Input: part model. Units: mm. Frame: model coordinates. A direction names the side the tool comes from. Give positions to 0.01 mm unless a question says otherwise; leave off trailing zeros. Loops run counter-clockwise (first coordinate to the right, second up) from the corner with the lowest first, then second, coordinate; pieces in that order, holes last. Notation, with made-up numbers: (-19.75, 53) -> (0.25, 53) arc R13 cw to (0.25, 62) -> close; hole circle Ø6 at (35.25, 51.5). An arc over 180 degrees is marked (long way). Answer as a JSON object with one key per item and string values.
```python
from build123d import *

# Parameters (mm, degrees)
F0_W     = 95
F0_H     = 90
F1_DEPTH = 20
F2_R     = 32.5
F3_DEPTH = 25
F4_R     = 17.5
F5_DEPTH = 25


with BuildPart() as f1:
    # F0 (on Top) → F1 (new body)
    with BuildSketch(Plane.XY):
        with Locations((-1.046643, 7.062163)):
            Rectangle(F0_W, F0_H)
        with BuildLine():
            ThreePointArc((46.453357, -37.937837), (91.453357, 7.062163), (46.453357, 52.062163))
            Line((46.453357, 52.062163), (46.453357, -37.937837))
        make_face()
    extrude(amount=F1_DEPTH)

    # F2 (on face) → F3 (join)
    with BuildSketch(Plane.XY.offset(20)):
        with Locations((46.453357, 7.062163)):
            Circle(F2_R)
    extrude(amount=F3_DEPTH)

    # F4 (on face) → F5 (cut)
    with BuildSketch(Plane.XY.offset(45)):
        with Locations((46.453357, 7.062163)):
            Circle(F4_R)
    extrude(amount=-F5_DEPTH, mode=Mode.SUBTRACT)


solid = f1.part
```
Q1. Section B-B, the plane x = 15.5. Return the cut outline in (y, z).
Evaluation:
{"outline": "(-37.94, 0) -> (52.06, 0) -> (52.06, 20) -> (16.97, 20) -> (16.97, 45) -> (-2.84, 45) -> (-2.84, 20) -> (-37.94, 20) -> close"}
Q2. Access query for faces 1 (the cylindrical face through (28.97, 7.83, 32.67)), 2 (the cylindrical face through (91.442, 6.073, 9.86)). Directions: +Z, -Z, +X, -X, +Y, -Y. A direction counts if a zero-diameter tool reaches every point of the face in a straight line with its end or side. Return the directions, or none.
Evaluation:
{"face 1": "+Z", "face 2": "+Z, -Z, +X"}
Q3. Section D-D, the plane z = 17.5. Return the cut outline in (x, y).
Evaluation:
{"outline": "(-48.55, -37.94) -> (46.45, -37.94) arc R45 ccw to (46.45, 52.06) -> (-48.55, 52.06) -> close"}
Q4. Pin query (flat end, axial travel): pin 1 (17.5 mm diameter, centred on x = 43.5, y = 3.5, fed in from +Z); pin 2 (1.5 mm diameter, centred on x = -26, z = 22, fed in from +Y); pin 3 (1 mm diameter, centred on x = 63, z = 24, fed in from -Y); pin 4 (2 mm diameter, centred on y = -1, z = 12.5, fed in from +X). Return the tip coordinate at first contact, or that it passes through.
Evaluation:
{"pin 1": "stops at z = 20", "pin 2": "passes through", "pin 3": "stops at y = -21.2", "pin 4": "stops at x = 90.9"}
Q5. Section A-A, the plane y = -18.5. Return the cut outline in (x, z).
Evaluation:
{"outline": "(-48.55, 0) -> (83.49, 0) -> (83.49, 20) -> (66.52, 20) -> (66.52, 45) -> (26.38, 45) -> (26.38, 20) -> (-48.55, 20) -> close"}
Q6. Ray query, line 1 along X through (y, z) = (7, 37); line 2 along Z through (x, y) = (46, 9); line 3 along Y through (x, z) = (44, 24.5). Return the intervals inside material, ascending.
Evaluation:
{"line 1": "x = 13.95 to 28.95, 63.95 to 78.95", "line 2": "z = 0 to 20", "line 3": "y = -25.35 to -10.27, 24.39 to 39.47"}
Q7. Draft query along Y for faces 3 (the cylindrical face through (77.453, 16.824, 32.325)), 4 (the flat face through (-2, -37.938, 10)), 5 (the flat face through (20, 8, 0)), 6 (the flat face through (46, 7, 20)). Return one class per face: +Y half, -Y half, draft (parallel to the pull), parting line (faces both ways), or undercut.
Evaluation:
{"face 3": "parting line", "face 4": "-Y half", "face 5": "draft", "face 6": "undercut"}
Q8. Section C-C, the plane z = 41. Return the cut outline in (x, y), then the cut area to 3 significant figures.
Evaluation:
{"outline": "circle Ø65 at (46.45, 7.06); hole circle Ø35 at (46.45, 7.06)", "area": "2,360 mm2"}
